Can you work these out from the drawing? Everything is in mm from the part's minimum corner. Give positions to 0.01 mm unless a question says otherwise; leave off trailing zeros. Order: outer loops, then holes, each group sorted by start corner. A loop starts at its lowest first (then second) coordinate and runs counter-clockwise, first axis right, second up. Notation, with made-up numbers: (-33.75, 50.5) - (24.25, 50.5) arc R10 cw to (24.25, 57.5) - close; hole circle Ø9 at (-40, 41). An arc over 180 degrees is marked (long way). One line per question, with ' | ' between items.
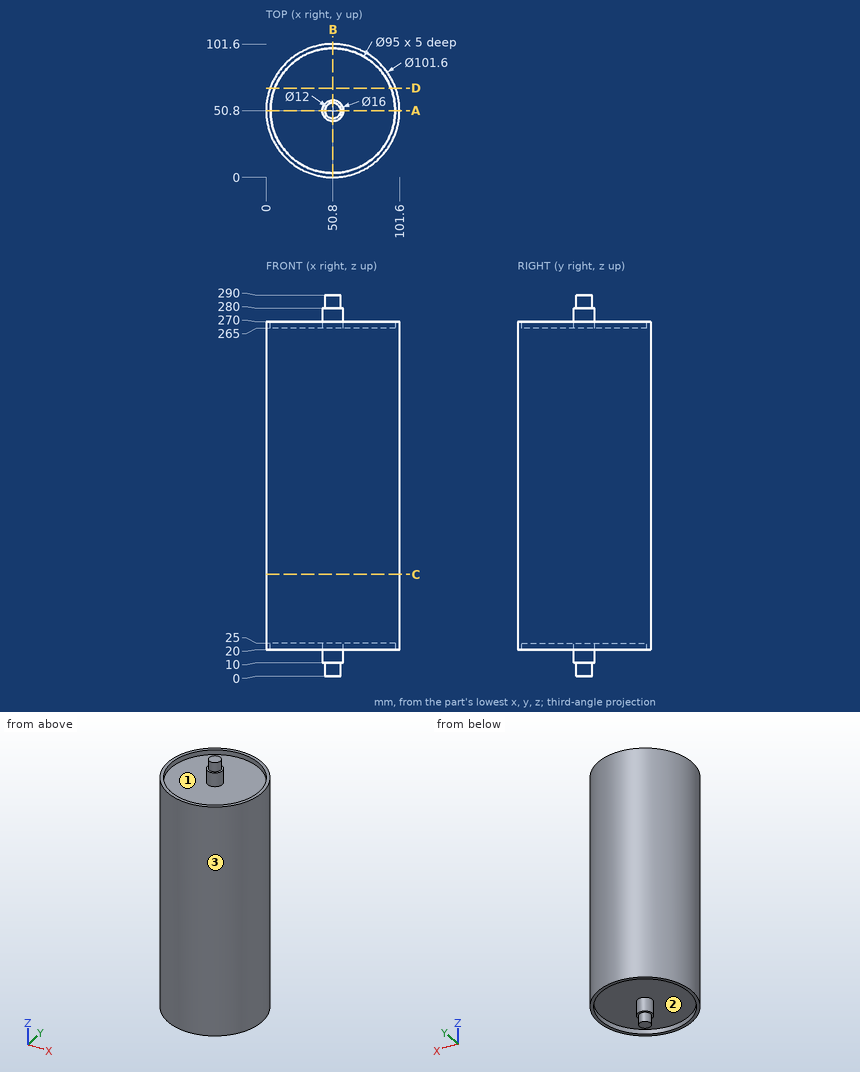
1) Thinking about a two-plate mould opening in X: for the marked faces 1, 2 and 3, which applies, +X half, -X half, draft (parallel to the pull), parting line (faces both ways), or undercut?
Model answer:
face 1: undercut | face 2: undercut | face 3: parting line
2) I want a section at D-D (y = 68). List the corners of the cut face in (x, z) for me, plus the area to 3 significant figures.
Model answer:
outline: (3, 20) - (6.52, 20) - (6.52, 25) - (95.08, 25) - (95.08, 20) - (98.6, 20) - (98.6, 270) - (95.08, 270) - (95.08, 265) - (6.52, 265) - (6.52, 270) - (3, 270) - close | area: 23,000 mm2
3) I want a section at C-C (z = 77.5). List the corners of the cut face in (x, y) for me, plus the area to 3 significant figures.
Model answer:
outline: circle Ø101.6 at (50.8, 50.8) | area: 8,110 mm2
4) I'm going to push flat-ended pins straight in: P1, Ø2, axis at x = 78.5, y = 20.5, coming from the +Z side; P2, Ø10, axis at y = 45.5, z = 74.5, coming from the +X side; P3, Ø3, axis at y = 88, z = 140, coming from the -X side. Where does each tip first touch, or does it pass through?
Model answer:
P1: stops at z = 265 | P2: stops at x = 101.6 | P3: stops at x = 14.66
5) Please list where these lines run through material, in increasing order: L1, parallel to Y at x = 50.8, z = 267.35; L2, parallel to Z at x = 76, y = 65; L3, parallel to Y at x = 60.5, z = 266.
Model answer:
L1: y = 0 to 3.3, 42.8 to 58.8, 98.3 to 101.6 | L2: z = 25 to 265 | L3: y = 0.93 to 4.3, 97.3 to 100.67
6) I want a section at A-A (y = 50.8). List the corners of the cut face in (x, z) for me.
Model answer:
outline: (0, 20) - (3.3, 20) - (3.3, 25) - (42.8, 25) - (42.8, 10) - (44.8, 10) - (44.8, 0) - (56.8, 0) - (56.8, 10) - (58.8, 10) - (58.8, 25) - (98.3, 25) - (98.3, 20) - (101.6, 20) - (101.6, 270) - (98.3, 270) - (98.3, 265) - (58.8, 265) - (58.8, 280) - (56.8, 280) - (56.8, 290) - (44.8, 290) - (44.8, 280) - (42.8, 280) - (42.8, 265) - (3.3, 265) - (3.3, 270) - (0, 270) - close
